Could you check a few things on this model? Use its own coordinates, in mm. A direction names the side the tool comes from. Round coordinates to 2 decimals unless told otherwise and drop trailing zeros. Loops run counter-clockwise (first coordinate to the right, second up) from the corner with the lowest first, then second, coordinate; pieces in that order, holes last. Notation, with made-up numbers: (20, 11.25) - (64, 11.25) arc R21 cw to (64, 31.25) - close; hole circle Ø2 at (45, -37.5). An arc over 180 degrees is marked (long way). Use one line per item in the form item = value.
```python
from build123d import *

# Parameters (mm, degrees)
F1_DEPTH = 2


with BuildPart() as f1:
    # F0 (on Right) → F1 (new body)
    with BuildSketch(Plane.YZ):
        with BuildLine():
            ThreePointArc((-16.050784, 75.634497), (-18.172104, 74.755817), (-19.050784, 72.634497))
            Line((-19.050784, 72.634497), (-19.050784, -21.365503))
            ThreePointArc((-19.050784, -21.365503), (-18.172104, -23.486823), (-16.050784, -24.365503))
            Line((-16.050784, -24.365503), (9, -24.365503))
            ThreePointArc((9, -24.365503), (11.12132, -23.486823), (12, -21.365503))
            Line((12, -21.365503), (12, 72.634497))
            ThreePointArc((12, 72.634497), (11.12132, 74.755817), (9, 75.634497))
            Line((9, 75.634497), (3, 75.634497))
            ThreePointArc((3, 75.634497), (0.87868, 74.755817), (0, 72.634497))
            Line((0, 72.634497), (0, -7.707447))
            ThreePointArc((0, -7.707447), (-0.87868, -9.828767), (-3, -10.707447))
            Line((-3, -10.707447), (-4.050784, -10.707447))
            ThreePointArc((-4.050784, -10.707447), (-6.172104, -9.828767), (-7.050784, -7.707447))
            Line((-7.050784, -7.707447), (-7.050784, 72.634497))
            ThreePointArc((-7.050784, 72.634497), (-7.929464, 74.755817), (-10.050784, 75.634497))
            Line((-10.050784, 75.634497), (-16.050784, 75.634497))
        make_face()
    extrude(amount=F1_DEPTH)


solid = f1.part
```
1. If we section it at A-A, the plane z = -2.5: Write out the boundary of the cut face in (x, y).
Solution:
outline = (0, -19.05) - (2, -19.05) - (2, -7.05) - (0, -7.05) - close; (0, 0) - (2, 0) - (2, 12) - (0, 12) - close
2. If we section it at B-B, the plane x = 0.65: Write out the boundary of the cut face in (y, z).
Solution:
outline = (-19.05, -21.37) arc R3 ccw to (-16.05, -24.37) - (9, -24.37) arc R3 ccw to (12, -21.37) - (12, 72.63) arc R3 ccw to (9, 75.63) - (3, 75.63) arc R3 ccw to (0, 72.63) - (0, -7.71) arc R3 cw to (-3, -10.71) - (-4.05, -10.71) arc R3 cw to (-7.05, -7.71) - (-7.05, 72.63) arc R3 ccw to (-10.05, 75.63) - (-16.05, 75.63) arc R3 ccw to (-19.05, 72.63) - close
3. Please list where these lines run through material, in increasing order: line 1 along Y through (x, z) = (1.2, -3.5); line 2 along Z through (x, y) = (0.2, 11); line 3 along Z through (x, y) = (0.9, -1).
Solution:
line_1 = -19.05 to -7.05, 0 to 12
line_2 = -23.6 to 74.87
line_3 = -24.37 to -9.94
4. If we section it at C-C, the plane y = -5: Write out the boundary of the cut face in (x, z), plus the area to 3 significant figures.
Solution:
outline = (0, -24.37) - (2, -24.37) - (2, -10.55) - (0, -10.55) - close
area = 27.6 mm^2
5. For P1, Ø6, axis at y = -3.5, z = 4.5, coming from the -X side, with a flat end and sliding along its axis, tell me the tip position at first contact or that it passes through.
Solution:
P1 = through
6. We'd pull the mould along Y, two halves only. Please class faces 3 (the face through (0.99, 11.1, -23.51)), 4 (the face through (1, -19.051, 26)), 5 (the face through (1, 6, 75.634)), 6 (the face through (0.986, 0.902, 74.779)): +Y half, -Y half, draft (parallel to the pull), parting line (faces both ways), or undercut.
Solution:
face_3 = +Y half
face_4 = -Y half
face_5 = draft
face_6 = undercut
7. On a 3-axis mill with a long thin cutter (end or side, diameter ignored), from which of +Z, -Z, +X, -X, +Y, -Y can I reach the whole of each face in a straight line? I mean faces 1 (the face through (1, 0, 33)), 2 (the face through (1, -13, 75.634)). Say none if no direction works.
Solution:
face_1 = +Z, +X, -X
face_2 = +Z, +X, -X, +Y, -Y
